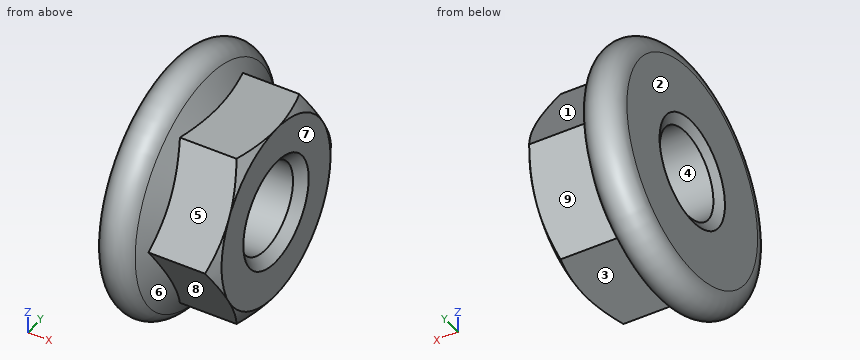
Autodesk Inventor part; units mm, degrees
ref_plane "Work Plane1" through (20.959, 0, 0) normal (0, 0, -1) x (-1, 0, 0)
ref_plane "YZ Plane" through (0, 0, 0) normal (1, 0, 0) x (0, 1, 0)
ref_plane "XZ Plane" through (0, 0, 0) normal (0, 1, 0) x (-1, 0, 0)
sketch "Sketch1" plane through (0, 0, 0) normal (0, 0, 1) x (1, 0, 0)
  line L0 (-1.4239, 0) -> (7.2373, 0)
  line L1 (2.78, 5) -> (2.0969, 6.4649)
  line L2 (2.78, 5) -> (6, 5) construction
  line L3 (6, 5) -> (6, 0) construction
  arc A0 (2.0969, 6.4649) -> (0, 6) centre (1.1, 6) ccw
  line L4 (2.78, 5) -> (2.78, 0)
  line L5 (0, -1.4613) -> (0, 8.7676)
  point P0 (0, 0)
  dimension "d2" = 10
  dimension "d4" = 14.2
  dimension "d5" = 1.1
  dimension "d15" = 6
  dimension "d16" = 25
revolve "Ring" add sketch "Sketch1" angle 360 about axis through (-10, 0, 0) along (1, 0, 0)
sketch "Sketch2" plane through (0, 0, 0) normal (-1, 0, 0) x (0, 0, 1)
  circle A0 centre (0, 0) radius 4.9
  line L0 (-5, -2.8868) -> (-5, 2.8868)
  line L1 (-5, 2.8868) -> (0, 5.7735)
  line L2 (0, 5.7735) -> (5, 2.8868)
  line L3 (5, 2.8868) -> (5, -2.8868)
  line L4 (5, -2.8868) -> (0, -5.7735)
  line L5 (0, -5.7735) -> (-5, -2.8868)
  circle A1 centre (0, 0) radius 6
  dimension "d6" = 11.547
extrude "Body" add sketch "Sketch2" against normal blind 6 contours A0 | L0 L1 L2 L3 L4 L5
sketch "Sketch3" plane through (0, 0, 0) normal (0, 0, 1) x (1, 0, 0)
  line L0 (2.4193, 5.7735) -> (6, 5.7735)
  line L1 (6, 2.8868) -> (6, 5.7735)
  line L2 (0, -6) -> (0, 6)
  line L3 (-1.2, 0) -> (7.2, 0)
  line L4 (5.5534, 5.7735) -> (6, 5)
  dimension "d10" = 30
  dimension "d11" = 10
revolve "Chamfer1" cut sketch "Sketch3" angle 360 about axis through (-10, 0, 0) along (1, 0, 0)
sketch "Sketch4" plane through (0, 0, 0) normal (-1, 0, 0) x (0, 0, 1)
  circle A0 centre (0, 0) radius 6
hole "Thread" at (0, 0, 0) direction (1, 0, 0) diameter 4.917 end through all
chamfer "Chamfer2" distance 0.5413 angle 30 1 edges at (0, 0, -2.4585) measured on face at (0, 4.7554, -0.5774)
ref_plane "Work Plane1" through (20.959, 0, 0) normal (0, 0, -1) x (-1, 0, 0)
chamfer "Chamfer3" distance 0.5413 angle 45 1 edges at (6, 0, -2.4585)
equation "\"d2\" = SW"
equation "\"d4\" = LADI"
equation "\"d5\" = PHH"
equation "\"d15\" = KOH"
equation "\"d16\" = KEWI"
equation "\"d6\" = 1.1547 * SW"
equation "\"d7\" = KOH"
equation "\"d10\" = ANG1"
equation "\"d11\" = SW0"
equation "\"d12\" = -0.5 * GD1 + 0.5 * NND"
equation "\"d46\" = -0.5 * GD1 + 0.5 * NND"
equation "\"d51\" = -0.5 * GD1 + 0.5 * NND"
equation "\"ANG1\" = 30deg"
equation "\"KEWI\" = 25deg"
equation "\"NND\" = 6"
equation "\"LADI\" = 14.2"
equation "\"SW\" = 10"
equation "\"PHH\" = 1.1"
equation "\"KOH\" = NND"
equation "\"SW0\" = 10"
equation "\"d1\" = LADI"
equation "\"d3\" = PHH"
equation "\"GUL\" = 0.541266 * PTC"
equation "\"RR\" = PHH"
equation "\"THREADDIA\" = 6"
equation "\"TOA\" = 30deg"
equation "\"PTC\" = 1"
equation "\"GAL\" = 0.541266 * PTC"
equation "\"E0\" = 1.155 * SW"
properties part number "ISO 4161 - M6(1)" material "Stainless Steel"
For this review, take the finished solid that the model builds, in its own axes (mm). Face numbers are marked on the shaded views. A direction names the side the tool comes from. Give positions to 0.01 mm unless a question says otherwise; leave off trailing zeros. Loops run counter-clockwise (first coordinate to the right, second up) from the corner with the lowest first, then second, coordinate; pieces in that order, holes last. Notation, with made-up numbers: M 14,18 L 29,18 A20 cw 29,50 Z; hole C 0,-22.75 d6. An arc over 180 degrees is marked long. Put each result on its own line as item: value. Start each with the question number.
(1) The part is to be moulded in two halves that separate along Z. For the marked faces 1, 2, 3 and 4, say which applies: +Z half, -Z half, draft (parallel to the pull), parting line (faces both ways), or undercut.
(2) Add section B-B, the plane x = 0.5. Write out the cut boundary in (y, z), then the cut area to 3 significant figures.
(3) Machinability: for the marked faces 5, 6, 7, 8 and 9, which of the approach directions +Z, -Z, +X, -X, +Y, -Y give a long, thin tool a straight path to every point of the face, cutting with its end or side? Answer none if there is none.
(4) For pin 1 (1.1 mm diameter, centred on x = 5, y = -0.5, fed in from +Z); pin 2 (1.8 mm diameter, centred on x = 4, y = -1, fed in from -Z); pin 3 (2 mm diameter, centred on x = 3.5, y = 0, fed in from -Z), all flat-tipped, find the tip position at first contact; note any pin that passes through.
(5) Wall thickness on L1, parallel to Z at x = 3.3, y = 0; L2, parallel to Z at x = 2, y = 0; L3, parallel to Y at x = 2.15, z = 0: over which ranges is each line inside the solid? List them lowest first.
(6) Add section A-A, the plane x = 3.5. Write out the cut boundary in (y, z).
(7) Add section C-C, the plane x = 1.25. Write out the cut boundary in (y, z), then the cut area to 3 significant figures.
Result:
1. face 1: +Z half
1. face 2: draft
1. face 3: -Z half
1. face 4: undercut
2. outline: C 0,0 d13.84; hole C 0,0 d4.92
2. area: 132 mm^2
3. face 5: +Z, +X, -Y
3. face 6: +X
3. face 7: +Z, -Z, +X, +Y, -Y
3. face 8: -Z, +X, -Y
3. face 9: -Z, +X, +Y
4. pin 1: stops at z = 5
4. pin 2: stops at z = -5
4. pin 3: stops at z = -5.6
5. L1: z = -5 to -2.46, 2.46 to 5
5. L2: z = -6.63 to -2.46, 2.46 to 6.63
5. L3: y = -6.35 to -2.46, 2.46 to 6.35
6. outline: M -5.77,0 L -2.89,-5 L 2.89,-5 L 5.77,0 L 2.89,5 L -2.89,5 Z; hole C 0,0 d4.92
7. outline: C 0,0 d14.18; hole C 0,0 d4.92
7. area: 139 mm^2
